```python
from build123d import *

# Parameters (mm, degrees)
KEY_MAIN_EXTURSION_DEPTH = 70
KEY_HANDLE_DEPTH         = 30
KEY_CUT_DEPTH            = 74.277343039


with BuildPart() as part:
    # Szkic1 → key-main-extursion (new body)
    with BuildSketch(Plane.XY):
        with BuildLine():
            Line((-1.381684649, -3.928424018), (-1.381684649, 4.071575982))
            Line((-1.381684649, 4.071575982), (-0.381684649, 4.071575982))
            Line((-0.381684649, 4.071575982), (-0.381684649, 8.071575982))
            Line((-0.381684649, 8.071575982), (-1.381684649, 8.071575982))
            Line((-1.381684649, 8.071575982), (-1.381684649, 12.071575982))
            ThreePointArc((-1.381684649, 12.071575982), (1.118315351, 14.571575982), (3.618315351, 12.071575982))
            Line((3.618315351, 12.071575982), (5.618315351, 10.071575982))
            Line((5.618315351, 10.071575982), (5.618315351, 8.071575982))
            Line((5.618315351, 8.071575982), (3.618315351, 8.071575982))
            Line((3.618315351, 8.071575982), (3.618315351, 0.071575982))
            Line((3.618315351, 0.071575982), (2.618315351, 0.071575982))
            Line((2.618315351, 0.071575982), (2.618315351, -3.928424018))
            Line((2.618315351, -3.928424018), (3.618315351, -3.928424018))
            Line((3.618315351, -3.928424018), (3.618315351, -7.928424018))
            ThreePointArc((3.618315351, -7.928424018), (1.118315351, -10.428424018), (-1.381684649, -7.928424018))
            Line((-1.381684649, -7.928424018), (-3.381684649, -5.928424018))
            Line((-3.381684649, -5.928424018), (-3.381684649, -3.928424018))
            Line((-3.381684649, -3.928424018), (-1.381684649, -3.928424018))
        make_face()
    extrude(amount=-KEY_MAIN_EXTURSION_DEPTH)

    # key-handle-sketch → key-handle (add)
    with BuildSketch(Plane.XY):
        with BuildLine():
            Line((-4.881684649, -9.253034266), (-4.881684649, 12.746965734))
            ThreePointArc((-4.881684649, 12.746965734), (1.118315351, 18.746965734), (7.118315351, 12.746965734))
            Line((7.118315351, 12.746965734), (7.118315351, -9.253034266))
            ThreePointArc((7.118315351, -9.253034266), (1.118315351, -15.253034266), (-4.881684649, -9.253034266))
        make_face()
    extrude(amount=KEY_HANDLE_DEPTH)

    # Szkic5 → key-cut (cut, through all)
    with BuildSketch(Plane.ZY.offset(3.75)):
        Polygon((-9.671572875, 14.571575982), (-15.328427125, 14.571575982), (-12.5, 11.743148857), align=None)
        Polygon((-15.580582618, 14.571575982), (-24.419417382, 14.571575982), (-20, 10.1521586), align=None)
        Polygon((-26.085786438, 14.571575982), (-28.914213562, 14.571575982), (-27.5, 13.15736242), align=None)
        Polygon((-30.050252532, 14.571575982), (-39.949747468, 14.571575982), (-35, 9.621828514), align=None)
        Polygon((-40.909009742, 14.571575982), (-44.090990258, 14.571575982), (-42.5, 12.980585724), align=None)
        Polygon((-46.464466094, 14.571575982), (-53.535533906, 14.571575982), (-50, 11.036042076), align=None)
        Polygon((-55.025126266, 14.571575982), (-59.974873734, 14.571575982), (-57.5, 12.096702248), align=None)
        Polygon((-61.641242789, 14.571575982), (-68.358757211, 14.571575982), (-65, 11.212818771), align=None)
        Polygon((-68.358757211, 14.571575982), (-70, 14.571575982), (-70, 12.930333193), align=None)
        Polygon((-70, -8.787181229), (-70, -10.428424018), (-68.358757211, -10.428424018), align=None)
        Polygon((-12.5, -7.599996893), (-15.328427125, -10.428424018), (-9.671572875, -10.428424018), align=None)
        Polygon((-20, -6.009006636), (-24.419417382, -10.428424018), (-15.580582618, -10.428424018), align=None)
        Polygon((-27.5, -9.014210456), (-28.914213562, -10.428424018), (-26.085786438, -10.428424018), align=None)
        Polygon((-35, -5.47867655), (-39.949747468, -10.428424018), (-30.050252532, -10.428424018), align=None)
        Polygon((-42.5, -8.83743376), (-44.090990258, -10.428424018), (-40.909009742, -10.428424018), align=None)
        Polygon((-50, -6.892890112), (-53.535533906, -10.428424018), (-46.464466094, -10.428424018), align=None)
        Polygon((-57.5, -7.953550284), (-59.974873734, -10.428424018), (-55.025126266, -10.428424018), align=None)
        Polygon((-65, -7.069666807), (-68.358757211, -10.428424018), (-61.641242789, -10.428424018), align=None)
    extrude(amount=-KEY_CUT_DEPTH, mode=Mode.SUBTRACT)


solid = part.part
```
Here's how the part is built. I have some questions about the finished solid (model axes, mm). A direction names the side the tool comes from. Round coordinates to 2 decimals unless told otherwise and drop trailing zeros. Order: outer loops, then holes, each group sorted by start corner. A loop starts at its lowest first (then second) coordinate and runs counter-clockwise, first axis right, second up. Notation, with made-up numbers: (46, 73) -> (86, 73) arc R10 cw to (86, 79) -> close; hole circle Ø11 at (32, -22). An arc over 180 degrees is marked (long way). Use a Markdown table: item, result. Add a question column.
(1) For faces 1 (the face through (1.3, -8.35, -66.28)), 2 (the face through (1.51, 12.54, -66.33)), 3 (the face through (-1.382, 9.6, -34.5)), which set-ups out of +Z, -Z, +X, -X, +Y, -Y let a thin tool reach every point of the face, with its end or its side?
(2) For pin 1 Ø3 at (y, z) = (-2.5, -18) entering from +X; pin 2 Ø0.6 at (x, z) = (4.5, -35) entering from -Y; pin 3 Ø1.1 at (x, z) = (3.5, -40) entering from -Y, each with a flat end and sliding along its axis, tell me the tip position at first contact or that it passes through.
(3) Suppose I cut it at A-A, the plane y = 6. Please give me the cut outline in (x, z).
(4) Suppose I cut it at D-D, the plane z = 6.5. Please give me the cut outline in (x, y), and give its area (3 significant figures).
(5) I need wall thicknesses on line 1 along Z through (x, y) = (-3.5, 7); line 2 along X through (y, z) = (-1, -36); line 3 along Y through (x, z) = (5, -35). Which ranges of each line are inside material? Lowest first, please.
(6) Suppose I cut it at C-C, the plane y = 1. Please give me the cut outline in (x, z).
(7) Suppose I cut it at B-B, the plane z = -45.5. Please give me the cut outline in (x, y), and give its area (3 significant figures).
(8) If we mould it in two halves opening along Y, with no side actions, what happens to faces 4 (the face through (0.85, -7.44, -33.04)), 5 (the face through (5.618, 9, -35)), 6 (the face through (2.618, -2, -35))? For each: released by +Y, released by -Y, zero draft, split by the parting line, or undercut.
Verdict:
| question | item | result |
|---|---|---|
| 1 | face 1 | +X, -X, -Y |
| 1 | face 2 | +X, -X, +Y |
| 1 | face 3 | -Z, -X, +Y |
| 2 | pin 1 | x = 3.62 |
| 2 | pin 2 | y = 8.07 |
| 2 | pin 3 | y = -9.63 |
| 3 | outline | (-4.88, 0) -> (-0.38, 0) -> (-0.38, -70) -> (3.62, -70) -> (3.62, 0) -> (7.12, 0) -> (7.12, 30) -> (-4.88, 30) -> close |
| 4 | outline | (-4.88, -9.25) arc R6 ccw to (7.12, -9.25) -> (7.12, 12.75) arc R6 ccw to (-4.88, 12.75) -> close |
| 4 | area | 377 mm2 |
| 5 | line 1 | 0 to 30 |
| 5 | line 2 | -1.38 to 2.62 |
| 5 | line 3 | 8.07 to 9.62 |
| 6 | outline | (-4.88, 0) -> (-1.38, 0) -> (-1.38, -70) -> (3.62, -70) -> (3.62, 0) -> (7.12, 0) -> (7.12, 30) -> (-4.88, 30) -> close |
| 7 | outline | (-3.38, -5.93) -> (-1.38, -7.93) arc R2.5 ccw to (3.62, -7.93) -> (3.62, -3.93) -> (2.62, -3.93) -> (2.62, 0.07) -> (3.62, 0.07) -> (3.62, 8.07) -> (5.62, 8.07) -> (5.62, 10.07) -> (3.62, 12.07) arc R2.5 ccw to (-1.38, 12.07) -> (-1.38, 8.07) -> (-0.38, 8.07) -> (-0.38, 4.07) -> (-1.38, 4.07) -> (-1.38, -3.93) -> (-3.38, -3.93) -> close |
| 7 | area | 124 mm2 |
| 8 | face 4 | released by -Y |
| 8 | face 5 | zero draft |
| 8 | face 6 | undercut |
